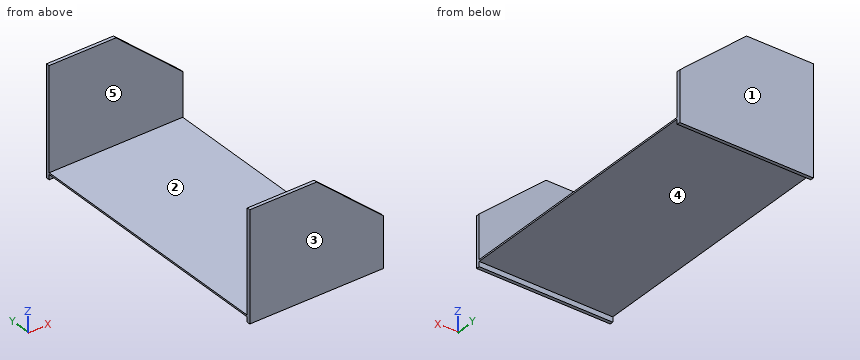
```python
from build123d import *

# Parameters (mm, degrees)
F0_W     = 101.6
F0_H     = 203.2
F1_DEPTH = 50.8
F3_DEPTH = 203.201
F4_W     = 198.12
F4_H     = 33.0125290838
F4_H_2   = 3.81
F5_W     = 67.5063457778
F5_H     = 198.12
F6_DEPTH = 101.601


with BuildPart() as f1:
    # F0 (on Top) → F1 (new body, symmetric)
    with BuildSketch(Plane.XY):
        Rectangle(F0_W, F0_H)
    extrude(amount=F1_DEPTH, both=True)

    # F2 (on face) → F3 (cut, through all)
    with BuildSketch(Plane.XZ.offset(101.6)):
        Polygon((-50.8, 50.8), (-50.8, 31.75), (0, 31.75), (50.8, -12.7074709162), (50.8, 50.8), align=None)
    extrude(amount=-F3_DEPTH, mode=Mode.SUBTRACT)

    # F4 (on face) + F5 (on face) → F6 (cut, through all)
    with BuildSketch(Plane.YZ.offset(50.8)):
        with Locations((0, -29.2137354581)):
            Rectangle(F4_W, F4_H)
        with Locations((0, -48.895)):
            Rectangle(F4_W, F4_H_2)
    with BuildSketch(Plane(origin=(15.7348640799, 0, 17.9796798779), x_dir=(0.7525218469, 0, -0.6585672858), z_dir=(0.6585672858, 0, 0.7525218469))):
        with Locations((12.8436615633, 0)):
            Rectangle(F5_W, F5_H)
    extrude(amount=-F6_DEPTH, dir=(1, 0, 0), mode=Mode.SUBTRACT)


solid = f1.part
```
Geometry: final body of the model. Coordinates: model frame, mm. Face numbers are marked on the shaded views. A direction names the side the tool comes from. Round coordinates to 2 decimals unless told otherwise and drop trailing zeros. Order: outer loops, then holes, each group sorted by start corner. A loop starts at its lowest first (then second) coordinate and runs counter-clockwise, first axis right, second up. Notation, with made-up numbers: (-5, -16.5) -> (10, -16.5) arc R14 cw to (10, -10.5) -> close; hole circle Ø6 at (-14, 33). An arc over 180 degrees is marked (long way). Write each question's results on one line, items separated by ' | '.
Q1. Section query B-B (x = -35.5). Output: boundary loops of the cut face in (y, z).
Response values:
outline: (-101.6, -50.8) -> (-99.06, -50.8) -> (-99.06, -46.99) -> (99.06, -46.99) -> (99.06, -50.8) -> (101.6, -50.8) -> (101.6, 31.75) -> (99.06, 31.75) -> (99.06, -45.72) -> (-99.06, -45.72) -> (-99.06, 31.75) -> (-101.6, 31.75) -> close
Q2. Section query A-A (z = -30.5). Output: boundary loops of the cut face in (x, y), and give its area (3 significant figures).
Response values:
outline: (-50.8, -101.6) -> (50.8, -101.6) -> (50.8, -99.06) -> (-50.8, -99.06) -> close; (-50.8, 99.06) -> (50.8, 99.06) -> (50.8, 101.6) -> (-50.8, 101.6) -> close | area: 516 mm²
Q3. Section query D-D (y = -34). Output: boundary loops of the cut face in (x, z), and give its area (3 significant figures).
Response values:
outline: (-50.8, -46.99) -> (50.8, -46.99) -> (50.8, -45.72) -> (-50.8, -45.72) -> close | area: 129 mm²
Q4. Pin query (flat end, axial travel): pin 1 Ø1 at (x, y) = (16, 33) entering from -Z; pin 2 Ø5 at (x, y) = (-35, 61) entering from +Z. Return the tip coordinate at first contact, or that it passes through.
Response values:
pin 1: z = -46.99 | pin 2: z = -45.72
Q5. Pull-direction query (Y, two-part tool) for the marked faces 1, 2 and 3; classes: released by +Y, released by -Y, zero draft, split by the parting line, or undercut.
Response values:
face 1: released by +Y | face 2: undercut | face 3: released by -Y
Q6. Access query for the marked faces 4 and 5. Directions: +Z, -Z, +X, -X, +Y, -Y. A direction counts if a zero-diameter tool reaches every point of the face in a straight line with its end or side. Return the directions, or none.
Response values:
face 4: -Z, +X, -X | face 5: +Z, +X, -X
Q7. Section query C-C (z = 5). Output: boundary loops of the cut face in (x, y).
Response values:
outline: (-50.8, -101.6) -> (30.57, -101.6) -> (30.57, -99.06) -> (-50.8, -99.06) -> close; (-50.8, 99.06) -> (30.57, 99.06) -> (30.57, 101.6) -> (-50.8, 101.6) -> close
Q8. Ray query, line 1 along Y through (x, z) = (-45.5, -40); line 2 along Z through (x, y) = (-25.5, -80). Return the intervals inside material, ascending.
Response values:
line 1: -101.6 to -99.06, 99.06 to 101.6 | line 2: -46.99 to -45.72
